Check sheet for the drawn part. Datum: minimum x, y, z corner. Units: mm. Round coordinates to 2 decimals unless told otherwise and drop trailing zeros. Write each loop counter-clockwise with the first axis right and the second up, starting at its lowest first coordinate (ties: lowest second). Pieces come first, ordered by that corner, then holes.
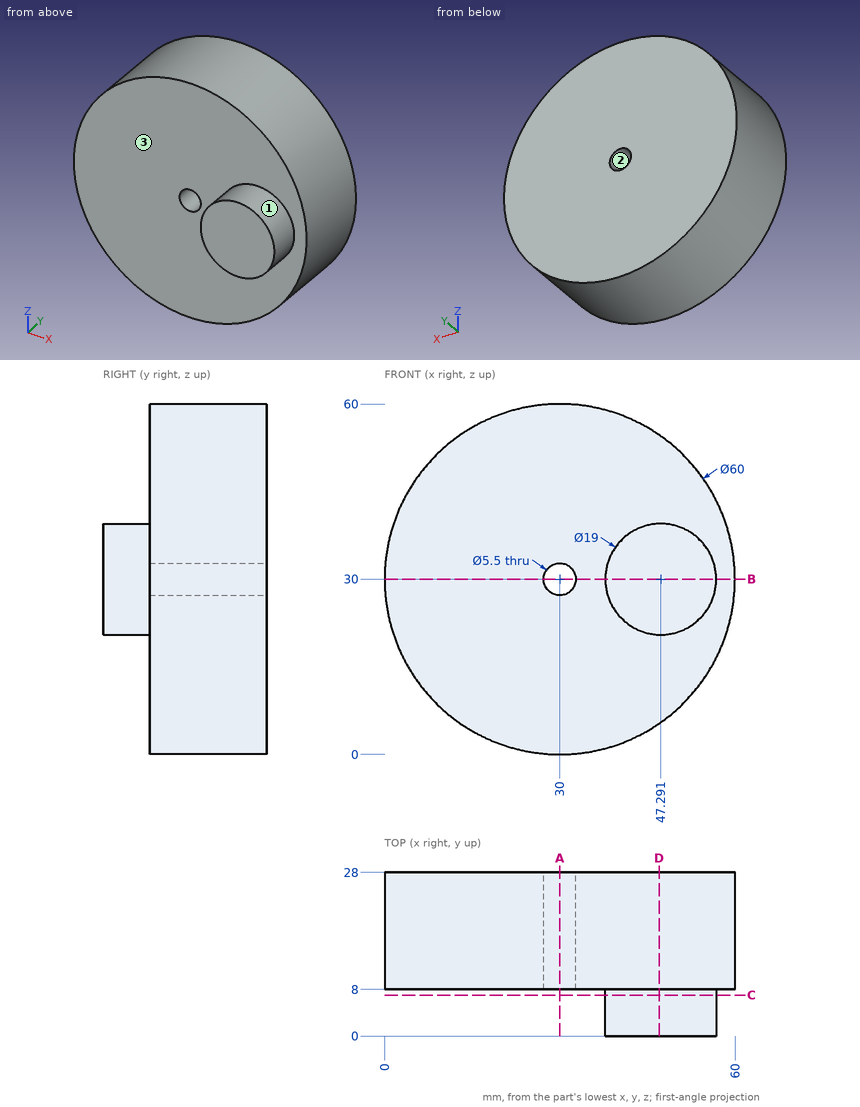
Q1. Sectioned sample at A-A (x = 30). Enter the section's corners in (y, z).
Recorded:
outline: (8, 0) - (28, 0) - (28, 27.25) - (8, 27.25) - close; (8, 32.75) - (28, 32.75) - (28, 60) - (8, 60) - close
Q2. Sectioned sample at B-B (z = 30). Enter the section's corners in (x, y), plus the area to 3 significant figures.
Recorded:
outline: (0, 8) - (27.25, 8) - (27.25, 28) - (0, 28) - close; (32.75, 8) - (37.79, 8) - (37.79, 0) - (56.79, 0) - (56.79, 8) - (60, 8) - (60, 28) - (32.75, 28) - close
area: 1,240 mm2
Q3. Sectioned sample at D-D (x = 47). Enter the section's corners in (y, z), plus the area to 3 significant figures.
Recorded:
outline: (0, 20.5) - (8, 20.5) - (8, 5.28) - (28, 5.28) - (28, 54.72) - (8, 54.72) - (8, 39.5) - (0, 39.5) - close
area: 1,140 mm2
Q4. Sectioned sample at C-C (y = 7). Enter the section's corners in (x, z).
Recorded:
outline: circle Ø19 at (47.29, 30)
Q5. Material ranges on line 1 along Z through (x, y) = (30, 18.75); line 2 along Y through (x, z) = (41.5, 22); line 3 along Z through (x, y) = (47.5, 1.75), recorded low to high.
Recorded:
line 1: z = 0 to 27.25, 32.75 to 60
line 2: y = 8 to 28
line 3: z = 20.5 to 39.5
Q6. Depth check by flat-ended pin: P1, Ø10, axis at x = 49.5, y = 17.5, coming from the +Z side; P2, Ø10, axis at x = 30, z = 48.5, coming from the -Y side; P3, Ø1, axis at x = 49, y = 22.5, coming from the -Z side. Enter the tip coordinate at first touch or a pass-through.
Recorded:
P1: stops at z = 56.26
P2: stops at y = 8
P3: stops at z = 6.38
Q7. Release check for a two-part mould opening along Z. For the marked faces 1, 2 and 3 record: released by +Z, released by -Z, zero draft, split by the parting line, or undercut.
Recorded:
face 1: split by the parting line
face 2: undercut
face 3: zero draft
